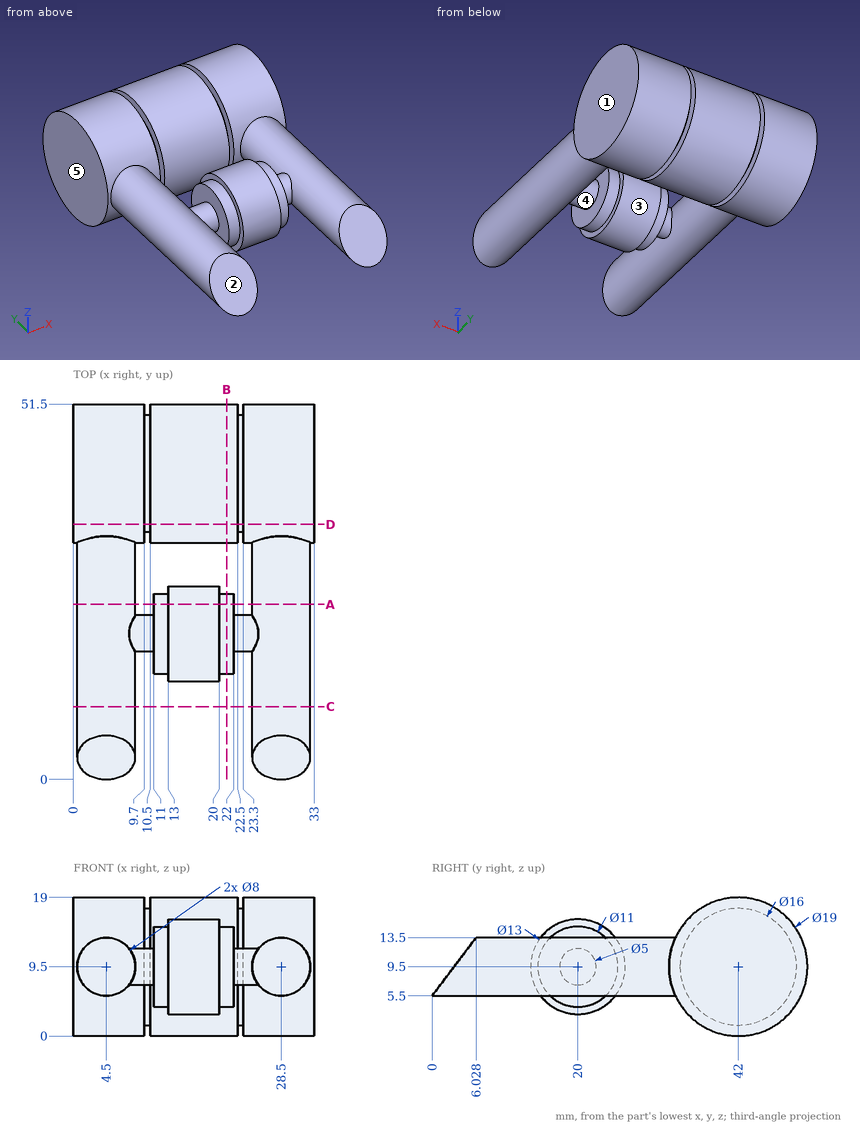
Here's the drawing with two shaded views (mm, measured from the low corner). I have some questions. A direction names the side the tool comes from. Give positions to 0.01 mm unless a question says otherwise; leave off trailing zeros. Write each loop counter-clockwise with the first axis right and the second up, starting at its lowest first coordinate (ties: lowest second). Pieces come first, ordered by that corner, then holes. Notation, with made-up numbers: (53, 11) -> (78, 11) arc R10 cw to (78, 29) -> close; hole circle Ø10 at (43.5, 14.25). An arc over 180 degrees is marked (long way). Answer as a JSON object with one key per item and string values. Group by question number.
Item 1: Suppose I cut it at B-B (x = 21). Please give me the cut outline in (y, z).
Item 2: Suppose I cut it at D-D (y = 35). Please give me the cut outline in (x, z).
Item 3: Suppose I cut it at A-A (y = 24). Please give me the cut outline in (x, z) (1 decimal).
Item 4: We'd pull the mould along X, two halves only. Please class the marked faces 1, 2 and 3: +X half, -X half, draft (parallel to the pull), parting line (faces both ways), or undercut.
Item 5: Suppose I cut it at C-C (y = 10). Please give me the cut outline in (x, z).
Item 6: For the marked faces 4 and 5, which set-ups out of +Z, -Z, +X, -X, +Y, -Y let a thin tool reach every point of the face, with its end or its side?
Item 7: I'm going to push flat-ended pins straight in: P1, Ø1.5, axis at x = 7.5, z = 7.5, coming from the -Y side (1 decimal); P2, Ø4, axis at y = 18, z = 8.5, coming from the +X side; P3, Ø10.5, axis at y = 20.5, z = 9.5, coming from the -X side; P4, Ø10, axis at x = 5, y = 44, coming from the +Z side. Where does each tip first touch, or does it pass through?
Item 8: Please list where these lines run through material, in increasing order: line 1 (X direction, y = 49, z = 14); line 2 (X direction, y = 12, z = 9.5); line 3 (Y direction, x = 21.5, z = 13). Write a range as [from, to].
Findings:
{
 "1": {"outline": "circle Ø11 at (20, 9.5); circle Ø19 at (42, 9.5)"},
 "2": {"outline": "(0, 3.08) -> (9.7, 3.08) -> (9.7, 5.63) -> (10.5, 5.63) -> (10.5, 3.08) -> (22.5, 3.08) -> (22.5, 5.63) -> (23.3, 5.63) -> (23.3, 3.08) -> (33, 3.08) -> (33, 15.92) -> (23.3, 15.92) -> (23.3, 13.37) -> (22.5, 13.37) -> (22.5, 15.92) -> (10.5, 15.92) -> (10.5, 13.37) -> (9.7, 13.37) -> (9.7, 15.92) -> (0, 15.92) -> close"},
 "3": {"outline": "circle Ø8 at (4.5, 9.5); (11, 5.7) -> (13, 5.7) -> (13, 4.4) -> (20, 4.4) -> (20, 5.7) -> (22, 5.7) -> (22, 13.3) -> (20, 13.3) -> (20, 14.6) -> (13, 14.6) -> (13, 13.3) -> (11, 13.3) -> close; circle Ø8 at (28.5, 9.5)"},
 "4": {"face 1": "+X half", "face 2": "draft", "face 3": "undercut"},
 "5": {"outline": "circle Ø8 at (4.5, 9.5); circle Ø8 at (28.5, 9.5)"},
 "6": {"face 4": "none", "face 5": "+Z, -Z, -X, +Y, -Y"},
 "7": {"P1": "stops at y = 0.9", "P2": "stops at x = 32.5", "P3": "stops at x = 0.5", "P4": "stops at z = 19"},
 "8": {"line 1": "x = [0, 9.7], [10.5, 22.5], [23.3, 33]", "line 2": "x = [0.5, 8.5], [24.5, 32.5]", "line 3": "y = [15.76, 24.24], [33.17, 50.83]"}
}
